from build123d import *

# Parameters (mm, degrees)
F0_W     = 457.2
F0_H     = 457.2
F1_DEPTH = 25.4
F0_W_2   = 203.2
F0_H_2   = 25.4
F2_DEPTH = 25.4
F0_W_3   = 76.2
F0_H_3   = 63.5
F3_DEPTH = 25.4


with BuildPart() as f1:
    # F0 (on Top) → F1 (new body)
    with BuildSketch(Plane.XY):
        with Locations((-163.00304, -103.314487)):
            Rectangle(F0_W, F0_H)
        Polygon((-290.00304, 99.885513), (-264.60304, 99.885513), (-61.40304, 99.885513), (-36.00304, 99.885513), (40.19696, 99.885513), (40.19696, -103.314487), (40.19696, -243.014487), (40.19696, -306.514487), (-36.00304, -306.514487), (-61.40304, -306.514487), (-264.60304, -306.514487), (-290.00304, -306.514487), (-366.20304, -306.514487), (-366.20304, -243.014487), (-366.20304, -103.314487), (-366.20304, 99.885513), align=None, mode=Mode.SUBTRACT)
    extrude(amount=F1_DEPTH)

    # F0 (on Top) → F2 (join)
    with BuildSketch(Plane.XY):
        Polygon((-264.60304, -77.914487), (-264.60304, 99.885513), (-290.00304, 99.885513), (-290.00304, -103.314487), (-290.00304, -243.014487), (-290.00304, -306.514487), (-264.60304, -306.514487), (-264.60304, -128.714487), (-264.60304, -103.314487), align=None)
        Polygon((-36.00304, 99.885513), (-61.40304, 99.885513), (-61.40304, -77.914487), (-61.40304, -103.314487), (-61.40304, -128.714487), (-61.40304, -306.514487), (-36.00304, -306.514487), (-36.00304, -243.014487), (-36.00304, -103.314487), align=None)
        with Locations((-163.00304, -116.014487)):
            Rectangle(F0_W_2, F0_H_2)
        with Locations((-163.00304, -90.614487)):
            Rectangle(F0_W_2, F0_H_2)
    extrude(amount=F2_DEPTH)

    # F0 (on Top) → F3 (join)
    with BuildSketch(Plane.XY):
        with Locations((-328.10304, -274.764487)):
            Rectangle(F0_W_3, F0_H_3)
        with Locations((2.09696, -274.764487)):
            Rectangle(F0_W_3, F0_H_3)
    extrude(amount=F3_DEPTH)


solid = f1.part
Source: CAD feature listing. Evaluate the final solid. Frame: model axes, mm. A direction names the side the tool comes from. Coordinates: 2 decimals unless noted, no trailing zeros. Loops run counter-clockwise (first coordinate to the right, second up) from the corner with the lowest first, then second, coordinate; pieces in that order, holes last. Notation, with made-up numbers: (83, 45) - (106, 45) arc R25 cw to (106, 60) - close; hole circle Ø1 at (78.25, 41.25). An arc over 180 degrees is marked (long way). One line per item, written item: value. Start each with the question number.
1. Section A-A (y = -287). Return the cut outline in (x, z), and give its area (3 significant figures).
2. Ray query, L1, parallel to X at y = -118.5, z = 15; L2, parallel to Y at x = -185, z = 11.5; L3, parallel to X at y = 72.5, z = 22. Return the intervals inside material, ascending.
3. Section B-B (x = -98). Return the cut outline in (y, z), and give its area (3 significant figures).
4. Set-up query: faces 1 (the flat face through (-391.603, -107, 13)), 2 (the flat face through (-61.403, 12, 13)). Return all of +Z, -Z, +X, -X, +Y, -Y with unobstructed straight access to the full face (end or side cutting, diameter ignored); none if empty.
5. Section C-C (x = -358). Return the cut outline in (y, z), and give its area (3 significant figures).
6. Mould query, pull axis Y, two halves, no side actions, for faces 3 (the flat face through (2, 99.886, 13)), 4 (the flat face through (-166, 125.286, 13)), 5 (the flat face through (-166, -331.914, 13)), 6 (the flat face through (-329, -243.014, 13)). Classes: pulls with the +Y half, pulls with the -Y half, needs draft (parallel to the pull), parting line crosses it, or undercut.
7. Section D-D (y = -199.5). Return the cut outline in (x, z).
Verdict:
1. outline: (-391.6, 0) - (-264.6, 0) - (-264.6, 25.4) - (-391.6, 25.4) - close; (-61.4, 0) - (65.6, 0) - (65.6, 25.4) - (-61.4, 25.4) - close
1. area: 6,450 mm2
2. L1: x = -391.6 to -366.2, -290 to -36, 40.2 to 65.6
2. L2: y = -331.91 to -306.51, -128.71 to -77.91, 99.89 to 125.29
2. L3: x = -391.6 to -366.2, -290 to -264.6, -61.4 to -36, 40.2 to 65.6
3. outline: (-331.91, 0) - (-306.51, 0) - (-306.51, 25.4) - (-331.91, 25.4) - close; (-128.71, 0) - (-77.91, 0) - (-77.91, 25.4) - (-128.71, 25.4) - close; (99.89, 0) - (125.29, 0) - (125.29, 25.4) - (99.89, 25.4) - close
3. area: 2,580 mm2
4. face 1: +Z, -Z, -X, +Y, -Y
4. face 2: +Z, -Z
5. outline: (-331.91, 0) - (-243.01, 0) - (-243.01, 25.4) - (-331.91, 25.4) - close; (99.89, 0) - (125.29, 0) - (125.29, 25.4) - (99.89, 25.4) - close
5. area: 2,900 mm2
6. face 3: undercut
6. face 4: pulls with the +Y half
6. face 5: pulls with the -Y half
6. face 6: undercut
7. outline: (-391.6, 0) - (-366.2, 0) - (-366.2, 25.4) - (-391.6, 25.4) - close; (-290, 0) - (-264.6, 0) - (-264.6, 25.4) - (-290, 25.4) - close; (-61.4, 0) - (-36, 0) - (-36, 25.4) - (-61.4, 25.4) - close; (40.2, 0) - (65.6, 0) - (65.6, 25.4) - (40.2, 25.4) - close
